```python
from build123d import *

# Parameters (mm, degrees)
SKETCH_1_W                                          = 24
SKETCH_1_H                                          = 24
SKETCH_1_R                                          = 1.7
WRIST_SPACER_W20_DEPTH                              = 20
GRIPPER_ADAPTER_M3_14X10_NOT_SG90_DIRECT_DEPTH      = 27.229754097
GRIPPER_ADAPTER_M3_14X10_NOT_SG90_DIRECT_DEPTH_BACK = 27.229754097
SKETCH_2_R                                          = 1.7


with BuildPart() as part:
    # 草图1 → Wrist_spacer_W20 (new body)
    with BuildSketch(Plane.XY):
        Rectangle(SKETCH_1_W, SKETCH_1_H)
        with Locations((-6, 0)):
            Circle(SKETCH_1_R, mode=Mode.SUBTRACT)
        with Locations((6, 0)):
            Circle(SKETCH_1_R, mode=Mode.SUBTRACT)
    extrude(amount=WRIST_SPACER_W20_DEPTH)

    # 草图2 → Gripper_adapter_M3_14x10_NOT_SG90_DIRECT (cut, two sides: drawn at the far end of the back side and taken through both)
    with BuildSketch(Plane(origin=(0, 0, 0), x_dir=(0, 0, -1), z_dir=(1, 0, 0)).offset(-GRIPPER_ADAPTER_M3_14X10_NOT_SG90_DIRECT_DEPTH_BACK)):
        with Locations((-5, -7)):
            Circle(SKETCH_2_R)
        with Locations((-15, -7)):
            Circle(SKETCH_2_R)
        with Locations((-5, 7)):
            Circle(SKETCH_2_R)
        with Locations((-15, 7)):
            Circle(SKETCH_2_R)
    extrude(amount=GRIPPER_ADAPTER_M3_14X10_NOT_SG90_DIRECT_DEPTH + GRIPPER_ADAPTER_M3_14X10_NOT_SG90_DIRECT_DEPTH_BACK, mode=Mode.SUBTRACT)


solid = part.part
```
Input: part model. Units: mm. Frame: model coordinates. Coordinates: 2 decimals unless noted, no trailing zeros. Write each loop counter-clockwise with the first axis right and the second up, starting at its lowest first coordinate (ties: lowest second). Pieces come first, ordered by that corner, then holes. Notation, with made-up numbers: (29, -23.5) -> (36, -23.5) arc R6 ccw to (36, -18.5) -> close; hole circle Ø4 at (83, 74). An arc over 180 degrees is marked (long way). Answer as a JSON object with one key per item and string values.
1. Section D-D on x = -0.25. Return the cut outline in (y, z), then the cut area to 3 significant figures.
Result set:
{"outline": "(-12, 0) -> (12, 0) -> (12, 20) -> (-12, 20) -> close; hole circle Ø3.4 at (-7, 5); hole circle Ø3.4 at (-7, 15); hole circle Ø3.4 at (7, 5); hole circle Ø3.4 at (7, 15)", "area": "444 mm2"}
2. Section C-C on y = 0. Return the cut outline in (x, z).
Result set:
{"outline": "(-12, 0) -> (-7.7, 0) -> (-7.7, 20) -> (-12, 20) -> close; (-4.3, 0) -> (4.3, 0) -> (4.3, 20) -> (-4.3, 20) -> close; (7.7, 0) -> (12, 0) -> (12, 20) -> (7.7, 20) -> close"}
3. Section B-B on x = -6. Return the cut outline in (y, z).
Result set:
{"outline": "(-12, 0) -> (-1.7, 0) -> (-1.7, 20) -> (-12, 20) -> close; (1.7, 0) -> (12, 0) -> (12, 20) -> (1.7, 20) -> close; hole circle Ø3.4 at (-7, 5); hole circle Ø3.4 at (-7, 15); hole circle Ø3.4 at (7, 5); hole circle Ø3.4 at (7, 15)"}
4. Section A-A on z = 5. Return the cut outline in (x, y).
Result set:
{"outline": "(-12, -12) -> (12, -12) -> (12, -8.7) -> (-12, -8.7) -> close; (-12, -5.3) -> (12, -5.3) -> (12, 5.3) -> (-12, 5.3) -> close; (-12, 8.7) -> (12, 8.7) -> (12, 12) -> (-12, 12) -> close; hole circle Ø3.4 at (-6, 0); hole circle Ø3.4 at (6, 0)"}
5. Material intervals for line 1 (Y direction, x = 4, z = 15); line 2 (Z direction, x = -4.25, y = 7); line 3 (X direction, y = -0.25, z = 11.5), sorted ascending. Write a range as from..to.
Result set:
{"line 1": "y = -12..-8.7, -5.3..5.3, 8.7..12", "line 2": "z = 0..3.3, 6.7..13.3, 16.7..20", "line 3": "x = -12..-7.68, -4.32..4.32, 7.68..12"}
6. Mould query, pull axis Z, two halves, no side actions, for faces 1 (the face through (0, 12, 10)), 2 (the face through (0, 0, 20)), 3 (the face through (-0.2, -8.5, 14.2)). Classes: released by +Z, released by -Z, zero draft, split by the parting line, or undercut.
Result set:
{"face 1": "zero draft", "face 2": "released by +Z", "face 3": "undercut"}
